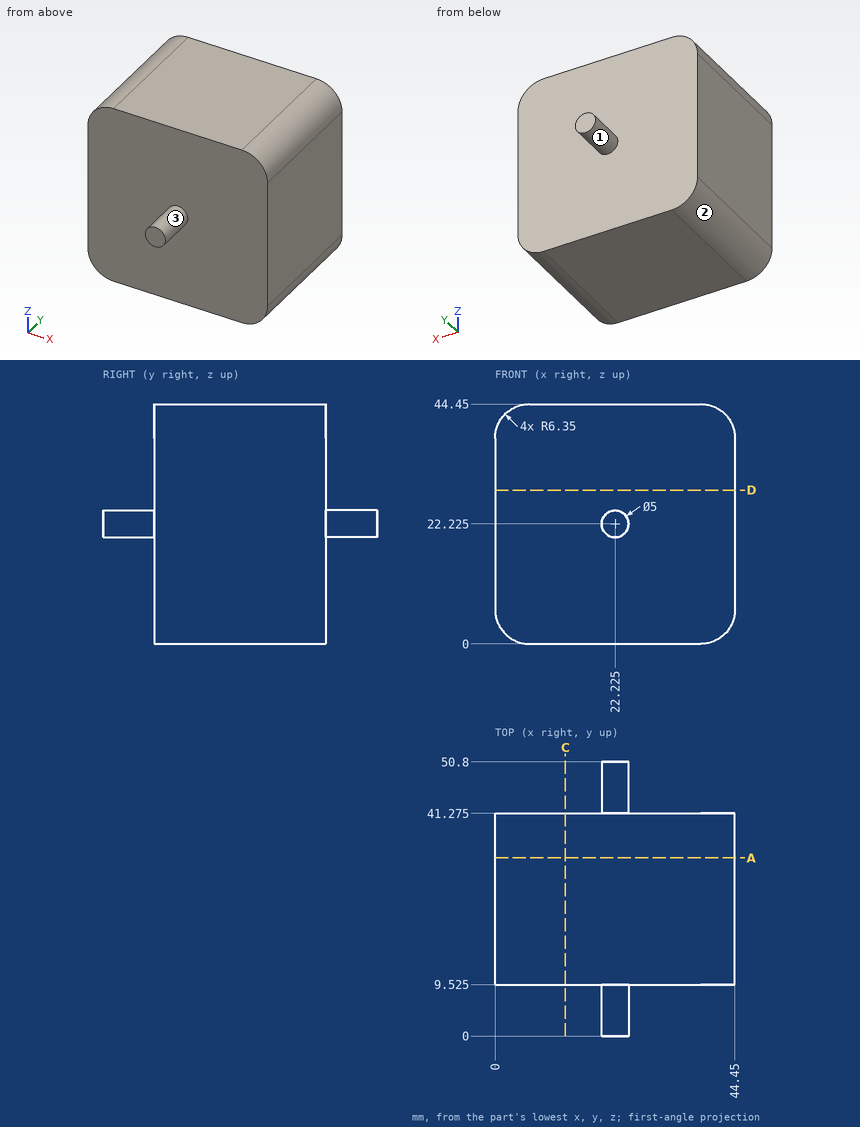
Can you work these out from the drawing? Everything is in mm from the part's minimum corner. A direction names the side the tool comes from. Round coordinates to 2 decimals unless told otherwise and drop trailing zeros. Write each loop counter-clockwise with the first axis right and the second up, starting at its lowest first coordinate (ties: lowest second). Pieces come first, ordered by that corner, then holes.
1. For the marked faces 1, 2 and 3, which set-ups out of +Z, -Z, +X, -X, +Y, -Y let a thin tool reach every point of the face, with its end or its side?
2. Suppose I cut it at D-D (z = 28.5). List the corners of the cut face in (x, y) for me (3 decimals).
3. Suppose I cut it at C-C (x = 13). List the corners of the cut face in (y, z) for me (3 decimals), and give its area (3 significant figures).
4. Suppose I cut it at A-A (y = 33). List the corners of the cut face in (x, z) for me.
5. Will these pins go through, and if not, where does the flat tip stop? pin 1 Ø8 at (x, z) = (8, 33) entering from -Y (3 decimals); pin 2 Ø6 at (x, z) = (10.5, 10.5) entering from +Y (3 decimals).
6. I need wall thicknesses on L1, parallel to Y at x = 39.5, z = 7.5 (3 decimals); L2, parallel to X at y = 41.5, z = 22; L3, parallel to X at y = 23, z = 40. Which ranges of each line are inside material? Lowest first, please.
Answer sheet:
1. face 1: +Y
1. face 2: -Z, -X, +Y, -Y
1. face 3: -Y
2. outline: (0, 9.525) - (44.45, 9.525) - (44.45, 41.275) - (0, 41.275) - close
3. outline: (9.525, 0) - (41.275, 0) - (41.275, 44.45) - (9.525, 44.45) - close
3. area: 1,410 mm2
4. outline: (0, 6.35) arc R6.35 ccw to (6.35, 0) - (38.1, 0) arc R6.35 ccw to (44.45, 6.35) - (44.45, 38.1) arc R6.35 ccw to (38.1, 44.45) - (6.35, 44.45) arc R6.35 ccw to (0, 38.1) - close
5. pin 1: stops at y = 9.525
5. pin 2: stops at y = 41.275
6. L1: y = 9.525 to 41.275
6. L2: x = 19.74 to 24.71
6. L3: x = 0.29 to 44.16
